Autodesk Inventor part; units mm, degrees
ref_plane "YZ Plane" through (0, 0, 0) normal (1, 0, 0) x (0, 1, 0)
ref_plane "XZ Plane" through (0, 0, 0) normal (0, 1, 0) x (-1, 0, 0)
ref_plane "XY Plane" through (0, 0, 0) normal (0, 0, 1) x (1, 0, 0)
sketch "Sketch1" plane through (0, 0, 0) normal (0, 0, 1) x (1, 0, 0)
  circle A0 centre (0, 0) radius 203.2
  circle A1 centre (0, 0) radius 127
  dimension "d0" = 406.4
  dimension "d1" = 76.2
extrude "Extrusion1" add sketch "Sketch1" along normal mid plane 152.4
chamfer "Chamfer1" distance 19.05 angle 45 2 edges at (-203.2, 0, 76.2) (-203.2, 0, -76.2)
fillet "Fillet2" radius 9.525 4 edges at (-203.2, 0, 57.15) (-184.15, 0, 76.2) (-203.2, 0, -57.15) (-184.15, 0, -76.2)
properties part number "tire"
Verification items for the finished model (mm, model axes). Coordinates: 2 decimals unless noted, no trailing zeros. Loops run counter-clockwise (first coordinate to the right, second up) from the corner with the lowest first, then second, coordinate; pieces in that order, holes last. Notation, with made-up numbers: (-13, 6.5) -> (25, 6.5) arc R31 ccw to (25, 30.5) -> close; hole circle Ø7 at (-2.5, 24). An arc over 180 degrees is marked (long way). Answer in a Markdown table with one row per item. Add a question column.
1. Material ranges on probe 1 along Y at (x, z) = (0, 30); probe 2 along X at (y, z) = (41, 41); probe 3 along Y at (x, z) = (61, 7), recorded low to high. Write a range as [from, to].
2. Depth check by flat-ended pin: P1, Ø8, axis at y = -151.5, z = -34, coming from the -X side; P2, Ø8, axis at y = 20, z = -16.5, coming from the +X side; P3, Ø12, axis at x = 139.5, z = 44, coming from the +Y side. Enter the tip coordinate at first touch or a pass-through.
3. Section check A-A, the plane z = 17. Enter the section's corners in (x, y).
4. Draft check along Y on faces 1 (the face through (-27.53, 123.98, -1.07)), 2 (the face through (-123, -38, -76.2)), 3 (the face through (-44.05, 198.368, -0.745)). Enter one of: +Y half, -Y half, draft (parallel to the pull), parting line (faces both ways), or undercut.
Derived:
| question | item | result |
|---|---|---|
| 1 | probe 1 | y = [-203.2, -127], [127, 203.2] |
| 1 | probe 2 | x = [-199.02, -120.2], [120.2, 199.02] |
| 1 | probe 3 | y = [-193.83, -111.39], [111.39, 193.83] |
| 2 | P1 | stops at x = -139.76 |
| 2 | P2 | stops at x = 202.57 |
| 2 | P3 | stops at y = 153.19 |
| 3 | outline | circle Ø406.4 at (0, 0); hole circle Ø254 at (0, 0) |
| 4 | face 1 | undercut |
| 4 | face 2 | draft |
| 4 | face 3 | parting line |
